Autodesk Inventor part; units mm, degrees
ref_plane "YZ Plane" through (0, 0, 0) normal (1, 0, 0) x (0, 1, 0)
ref_plane "XZ Plane" through (0, 0, 0) normal (0, 1, 0) x (-1, 0, 0)
ref_plane "XY Plane" through (0, 0, 0) normal (0, 0, 1) x (1, 0, 0)
sketch "스케치2" plane through (0, 0, 0) normal (0, 1, 0) x (-1, 0, 0)
  line L0 (49.375, -35.275) -> (-49.375, -35.275)
  line L1 (-49.375, -35.275) -> (-49.375, 35.275)
  line L2 (-49.375, 35.275) -> (49.375, 35.275)
  line L3 (49.375, 35.275) -> (49.375, -35.275)
  line L4 (49.375, -35.275) -> (-49.375, 35.275) construction
  line L5 (-49.375, -35.275) -> (49.375, 35.275) construction
  line L6 (54.375, -40.275) -> (-54.375, -40.275)
  line L7 (-54.375, -40.275) -> (-54.375, 40.275)
  line L8 (-54.375, 40.275) -> (54.375, 40.275)
  line L9 (54.375, 40.275) -> (54.375, -40.275)
  point P0 (0, 0)
  dimension "d0" = 98.75
  dimension "d1" = 70.55
  dimension "d2" = 5
extrude "돌출1" add sketch "스케치2" along normal blind 30
sketch "스케치3" plane through (0, 0, 0) normal (0, 1, 0) x (-1, 0, 0)
  line L0 (54.375, 40.275) -> (-54.375, 40.275) construction
  line L1 (54.375, -40.275) -> (-54.375, -40.275)
  line L2 (-54.375, -40.275) -> (-54.375, 40.275)
  line L3 (-54.375, 40.275) -> (54.375, 40.275)
  line L4 (54.375, 40.275) -> (54.375, -40.275)
  line L5 (54.375, -40.275) -> (-54.375, 40.275) construction
  line L6 (-54.375, -40.275) -> (54.375, 40.275) construction
  point P0 (0, 0)
extrude "돌출2" add sketch "스케치3" against normal blind 5
sketch "스케치4" plane through (0, -5, 0) normal (0, -1, 0) x (1, 0, 0)
  line L0 (26.325, -26.325) -> (-26.325, -26.325)
  line L1 (-26.325, -26.325) -> (-26.325, 26.325)
  line L2 (-26.325, 26.325) -> (26.325, 26.325)
  line L3 (26.325, 26.325) -> (26.325, -26.325)
  line L4 (26.325, -26.325) -> (-26.325, 26.325) construction
  line L5 (-26.325, -26.325) -> (26.325, 26.325) construction
  line L6 (-26.325, 19.2539) -> (-19.2539, 26.325)
  line L7 (-19.2539, -26.325) -> (-26.325, -19.2539)
  line L8 (26.325, -19.2539) -> (19.2539, -26.325)
  line L9 (19.2539, 26.325) -> (26.325, 19.2539)
  point P0 (0, 0)
  dimension "d7" = 52.65
  dimension "d8" = 52.65
  dimension "d9" = 45
  dimension "d10" = 5
  dimension "d13" = 360
extrude "돌출3" cut sketch "스케치4" against normal through all contours L0 L7 L1 L6 L2 L9 L3 L8
sketch "스케치5" plane through (-54.375, 30, -40.275) normal (-1, 0, 0) x (0, 0, 1)
  line L0 (80.55, -35) -> (0, -35) construction
  circle A0 centre (40.275, -17.5) radius 1.5
  circle A1 centre (25.275, -17.5) radius 1.5
  circle A2 centre (55.275, -17.5) radius 1.5
  point P0 (40.275, -30)
  dimension "d17" = 3
  dimension "d18" = 17.5
  dimension "d19" = 3
  dimension "d20" = 17.5
  dimension "d21" = 17.5
  dimension "d22" = 3
  dimension "d23" = 15
  dimension "d24" = 0
  dimension "d25" = 15
extrude "돌출4" cut sketch "스케치5" against normal blind 5
fillet "모깎기1" radius 2.5 8 edges at (-54.375, 12.5, 40.275) (54.375, 12.5, 40.275) (54.375, 12.5, -40.275) (-54.375, 12.5, -40.275) (-54.375, -5, 0) (0, -5, -40.275) (0, -5, 40.275) (54.375, -5, 0)
chamfer "모따기1" distance 2 angle 45 11 edges at (-49.375, 12.5, 13.5) (-49.375, 12.5, -1.5) (-49.375, 12.5, -16.5) (0, -5, -26.325) (22.7895, -5, -22.7895) (26.325, -5, 0) (22.7895, -5, 22.7895) (0, -5, 26.325) (-22.7895, -5, 22.7895) (-26.325, -5, 0) (-22.7895, -5, -22.7895)
sketch "스케치6" plane through (0, -5, 0) normal (0, -1, 0) x (1, 0, 0)
  circle A0 centre (-40.35, 0) radius 6.6
  line L0 (-54.375, 37.775) -> (-54.375, -37.775) construction
  line L1 (-26.325, -19.2539) -> (-26.325, 19.2539) construction
  point P0 (0, 0)
  dimension "d32" = 13.2
  dimension "d33" = 14.025
  dimension "d34" = 14.025
extrude "돌출5" cut sketch "스케치6" against normal blind 5
chamfer "모따기2" distance 2 angle 45 1 edges at (-46.95, 0, 0)
sketch "스케치7" plane through (0, 30, 0) normal (0, 1, 0) x (1, 0, 0)
  line L0 (-54.375, 37.775) -> (-54.375, -37.775) construction
  line L1 (54.375, -37.775) -> (54.375, 37.775) construction
  line L2 (-49.375, 35.275) -> (49.375, 35.275) construction
  circle A0 centre (-51.875, 0) radius 1.5
  line L3 (-51.875, -37.775) -> (51.875, -37.775) construction
  circle A1 centre (0, -37.775) radius 1.5
  circle A2 centre (34.375, 37.775) radius 1.5
  point P0 (0, 0)
  dimension "d40" = 3
  dimension "d41" = 2.5
  dimension "d42" = 3
  dimension "d43" = 3
  dimension "d44" = 2.5
  dimension "d45" = 20
extrude "돌출6" cut sketch "스케치7" against normal blind 5
equation "\"d33\" = d34"
properties part number "housing_top"
Can you work these out from the model? Positions are in its coordinate system, mm. A direction names the side the tool comes from. Coordinates: 2 decimals unless noted, no trailing zeros. Write each loop counter-clockwise with the first axis right and the second up, starting at its lowest first coordinate (ties: lowest second). Pieces come first, ordered by that corner, then holes. Notation, with made-up numbers: (63, 71.25) - (119, 71.25) arc R31 ccw to (119, 103.25) - close; hole circle Ø1 at (51, 55.25). An arc over 180 degrees is marked (long way). Return JSON: item names as keys, results as strings.
Q1. If we section it at A-A (x = -40.35): Please give me the cut outline in (y, z) (3 decimals).
Computed values:
{"outline": "(-5, -37.775) arc R2.5 ccw to (-2.5, -40.275) - (30, -40.275) - (30, -35.275) - (0, -35.275) - (0, -8.6) - (-2, -6.6) - (-5, -6.6) - close; (-5, 6.6) - (-2, 6.6) - (0, 8.6) - (0, 35.275) - (30, 35.275) - (30, 40.275) - (-2.5, 40.275) arc R2.5 ccw to (-5, 37.775) - close"}
Q2. Please list where these lines run through material, in increasing order: L1, parallel to X at y = 27.9, z = 0 (3 decimals); L2, parallel to Z at x = 0, y = 26.9 (3 decimals); L3, parallel to Z at x = 20, y = 16.5 (3 decimals). Write a range as from..to.
Computed values:
{"L1": "x = -54.375..-53.375, -50.375..-49.375, 49.375..54.375", "L2": "z = -40.275..-35.275, 35.275..36.275, 39.275..40.275", "L3": "z = -40.275..-35.275, 35.275..40.275"}
Q3. On a 3-axis mill with a long thin cutter (end or side, diameter ignored), from which of +Z, -Z, +X, -X, +Y, -Y can I reach the whole of each face in a straight line? I mean faces 4 (the flat face through (0, 25, 38)), 5 (the conical face through (-51.25, 14.086, -0.352)), 6 (the flat face through (-23.429, -3.986, -23.544)), 7 (the cylindrical face through (-52.9, 12.57, 13.5)), 8 (the flat face through (0, -2, 26.325)). Say none if no direction works.
Computed values:
{"face 4": "+Y", "face 5": "none", "face 6": "-Y", "face 7": "-X", "face 8": "+Y, -Y"}
Q4. I'm going to push flat-ended pins straight in: pin 1 Ø2 at (x, z) = (-37, -12.5) entering from +Y; pin 2 Ø3 at (x, z) = (-0.5, 25) entering from -Y (3 decimals); pin 3 Ø2.5 at (y, z) = (12.5, 15) entering from -X (3 decimals). Where does each tip first touch, or does it pass through?
Computed values:
{"pin 1": "stops at y = 0", "pin 2": "stops at y = -3.175", "pin 3": "stops at x = 49.375"}
Q5. If we section it at C-C (z = 0): Count the separate pieces of the cut face and the enclosed holes in it, then the cut area to 3 significant figures.
Computed values:
{"separate pieces": "4", "enclosed holes": "0", "area": "470 mm2"}
Q6. If we section it at B-B (z = -15): Please give me the cut outline in (x, y) (3 decimals), then the cut area to 3 significant figures.
Computed values:
{"outline": "(-54.375, -2.5) arc R2.5 ccw to (-51.875, -5) - (-28.325, -5) - (-26.325, -3) - (-26.325, 0) - (-49.375, 0) - (-49.375, 9) - (-51.375, 11) - (-54.375, 11) - close; (-54.375, 14) - (-51.375, 14) - (-49.375, 16) - (-49.375, 30) - (-54.375, 30) - close; (26.325, -3) - (28.325, -5) - (51.875, -5) arc R2.5 ccw to (54.375, -2.5) - (54.375, 30) - (49.375, 30) - (49.375, 0) - (26.325, 0) - close", "area": "555 mm2"}
Q7. Thinking about a two-plate mould opening in X: for faces 1 (the flat face through (1, 14, 40.275)), 2 (the cylindrical face through (53.62, -4.29, 0.53)), 3 (the flat face through (49.375, 15, 0)), which applies, +X half, -X half, draft (parallel to the pull), parting line (faces both ways), or undercut?
Computed values:
{"face 1": "draft", "face 2": "+X half", "face 3": "undercut"}
